from build123d import *

# Parameters (mm, degrees)
SKETCH1_R                = 4
BOSS_EXTRUDE1_DEPTH      = 55
BOSS_EXTRUDE2_DEPTH      = 2
BOSS_EXTRUDE2_DEPTH_BACK = 2
SKETCH2_R                = 2.5
SKETCH3_R                = 5.5
BOSS_EXTRUDE3_DEPTH      = 3
CHAMFER1_SIZE            = 2
BOSS_EXTRUDE4_START      = 20
SKETCH4_R                = 4
BOSS_EXTRUDE4_DEPTH      = 20
SKETCH5_OUTSIDE_W        = 30.092
SKETCH5_OUTSIDE_H        = 30.092
SKETCH5_OUTSIDE_R        = 4
CUT_EXTRUDE1_DEPTH       = 85.393094269
CHAMFER2_SIZE            = 3
CHAMFER3_SIZE            = 3


with BuildPart() as part:
    # Sketch1 → Boss-Extrude1 (new body)
    with BuildSketch(Plane(origin=(0, 0, 0), x_dir=(1, 0, 0), z_dir=(0, 1, 0))):
        with Locations(Location((0, 0, 0), (0, 0, 270))):
            Circle(SKETCH1_R)
    extrude(amount=BOSS_EXTRUDE1_DEPTH)

    # Sketch2 → Boss-Extrude2 (add, two sides: drawn at the far end of the back side and taken through both)
    with BuildSketch(Plane(origin=(0, 0, 0), x_dir=(0, 0, -1), z_dir=(1, 0, 0)).offset(-BOSS_EXTRUDE2_DEPTH_BACK)):
        with BuildLine():
            Line((-4, 60.033888167), (-4, 55))
            Line((-4, 55), (4, 55))
            Line((4, 55), (4, 60.033888167))
            ThreePointArc((4, 60.033888167), (0, 64.033888167), (-4, 60.033888167))
        make_face()
        with Locations((0, 60.033888167)):
            Circle(SKETCH2_R, mode=Mode.SUBTRACT)
    extrude(amount=BOSS_EXTRUDE2_DEPTH + BOSS_EXTRUDE2_DEPTH_BACK)

    # Sketch3 → Boss-Extrude3 (add)
    with BuildSketch(Plane.XZ.offset(-55)):
        with Locations(Location((0, 0, 0), (0, 0, 270))):
            Circle(SKETCH3_R)
    extrude(amount=BOSS_EXTRUDE3_DEPTH)

    # Chamfer1
    # the kernel refuses this chamfer: 2 mm, written as the material it takes off along each edge
    with BuildSketch(Plane(origin=(0, 52, 0), x_dir=(0, 0, -1), z_dir=(-1, 0, 0))) as chamfer1_piece_1_section:
        Polygon((5.5 - CHAMFER1_SIZE, 0), (5.5, -CHAMFER1_SIZE), (5.5, 0), align=None)
    chamfer1_piece_1 = revolve(axis=Axis((0, 52, 0), (0, -1, 0)), mode=Mode.PRIVATE)
    chamfer1_piece_1 = chamfer1_piece_1 - Plane(origin=(0, 53.250152147, 0), x_dir=(0, 0, 1), z_dir=(0, -1, 0)) * Cylinder(4, 22, mode=Mode.PRIVATE)
    add(chamfer1_piece_1, mode=Mode.SUBTRACT)

    # Sketch4 → Boss-Extrude4 (add)
    with BuildSketch(Plane.XZ.offset(BOSS_EXTRUDE4_START)):
        with Locations(Location((0, 0, 0), (0, 0, 270))):
            Circle(SKETCH4_R)
    extrude(amount=-BOSS_EXTRUDE4_DEPTH)

    # Sketch5 outside → Cut-Extrude1 (cut, through all)
    with BuildSketch(Plane.XZ.offset(20)):
        Rectangle(SKETCH5_OUTSIDE_W, SKETCH5_OUTSIDE_H)
        with Locations(Location((0, 0, 0), (0, 0, 270))):
            Circle(SKETCH5_OUTSIDE_R, mode=Mode.SUBTRACT)
    extrude(amount=-CUT_EXTRUDE1_DEPTH, mode=Mode.SUBTRACT)

    # Chamfer2
    # the kernel refuses this chamfer: 3 mm, written as the material it takes off along each edge
    with BuildSketch(Plane(origin=(0, 55, 0), x_dir=(-0.9865404268898706, 0, -0.16351754068586014), z_dir=(-0.16351754068586014, 0, 0.9865404268898706))) as chamfer2_piece_1_section:
        Polygon((4, CHAMFER2_SIZE), (4 - CHAMFER2_SIZE, 0), (4, 0), align=None)
    chamfer2_piece_1 = revolve(axis=Axis((0, 55, 0), (0, -1, 0)), revolution_arc=341.177747572, mode=Mode.PRIVATE)
    chamfer2_piece_1 = split(chamfer2_piece_1, bisect_by=Plane(origin=(2, 53.817100825, 1e-09), z_dir=(1, 0, 0)), keep=Keep.TOP, mode=Mode.PRIVATE)
    add(chamfer2_piece_1, mode=Mode.SUBTRACT)

    # Chamfer3
    # the kernel refuses this chamfer: 3 mm, written as the material it takes off along each edge
    with BuildSketch(Plane(origin=(0, 55, 0), x_dir=(0.9865404268898706, 0, 0.16351754068586002), z_dir=(0.16351754068586002, 0, -0.9865404268898706))) as chamfer3_piece_1_section:
        Polygon((4, CHAMFER3_SIZE), (4 - CHAMFER3_SIZE, 0), (4, 0), align=None)
    chamfer3_piece_1 = revolve(axis=Axis((0, 55, 0), (0, -1, 0)), revolution_arc=341.177747572, mode=Mode.PRIVATE)
    chamfer3_piece_1 = split(chamfer3_piece_1, bisect_by=Plane(origin=(-2, 53.794161032, -4e-09), z_dir=(-1, 0, 0)), keep=Keep.TOP, mode=Mode.PRIVATE)
    add(chamfer3_piece_1, mode=Mode.SUBTRACT)


solid = part.part
Read the model definition and answer for the solid it produces. Units are mm, in the model's axes. Round coordinates to 2 decimals unless told otherwise and drop trailing zeros. Write each loop counter-clockwise with the first axis right and the second up, starting at its lowest first coordinate (ties: lowest second). Pieces come first, ordered by that corner, then holes.
Q1. Find section C-C on y = 23. Determine the outline of the cut face in (x, z).
Values:
outline: circle Ø8 at (0, 0)
Q2. Find section B-B on x = -1. Determine the outline of the cut face in (y, z).
Values:
outline: (-20, -3.87) - (61.03, -3.87) arc R4 ccw to (61.03, 3.87) - (-20, 3.87) - close; hole circle Ø5 at (60.03, 0)
Q3. The mould has two halves that part along Y. Classify faces 1 (the face through (-0.028, 57.593, 0.542)), 2 (the face through (0, -20, 0)), 3 (the face through (-0.028, 64.033, -0.088)): released by +Y, released by -Y, zero draft, split by the parting line, or undercut.
Values:
face 1: undercut
face 2: released by -Y
face 3: released by +Y
Q4. Straight lines are drawn through the part: line 1 (Z direction, x = -2, y = 25); line 2 (X direction, y = 56, z = 0.5); line 3 (Y direction, x = 1, z = -1.75). For each, find the intervals that lie inside material, in ascending order.
Values:
line 1: z = -3.46 to 3.46
line 2: x = -2 to 2
line 3: y = -20 to 58.25, 61.82 to 63.63
Q5. Flat-ended cylindrical pins translate along their axes: P1, Ø1, axis at x = 2, y = -4.5, coming from the +Z side; P2, Ø1.5, axis at x = 3, y = 52, coming from the -Z side; P3, Ø1.5, axis at y = 54, z = 1, coming from the -X side. Find the tip coordinate at first contact, or state that the pin passes through.
Values:
P1: stops at z = 3.71
P2: stops at z = -3.31
P3: stops at x = -2.6
Q6. Find section A-A on z = 0. Determine the outline of the cut face in (x, y), and give its area (3 significant figures).
Values:
outline: (-4, -20) - (4, -20) - (4, 52) - (2, 54) - (2, 57.53) - (-2, 57.53) - (-2, 54) - (-4, 52) - close; (-2, 62.53) - (2, 62.53) - (2, 64.03) - (-2, 64.03) - close
area: 608 mm2
